Read the model definition and answer for the solid it produces. Units are mm, in the model's axes. A direction names the side the tool comes from. Coordinates: 2 decimals unless noted, no trailing zeros. Loops run counter-clockwise (first coordinate to the right, second up) from the corner with the lowest first, then second, coordinate; pieces in that order, holes last.
Q1. The mould has two halves that part along X. Classify faces 6 (the face through (-38.966, -1.985, -0.521)), 7 (the face through (9.028, 35.796, -19.907)), 8 (the face through (0, 36, -28)): pulls with the +X half, pulls with the -X half, needs draft (parallel to the pull), parting line crosses it, or undercut.
Q2. Section C-C (y = 30) is taken. Give the vertices of the cut face in (x, z), then the cut area to 3 significant figures.
Q3. Straight lines are drawn through the part: line 1 (X direction, y = -5.5, z = 0); line 2 (Y direction, x = 3, z = 23.5); line 3 (Z direction, x = 0, y = 7). For each, find the intervals that lie inside material, in ascending order.
Q4. Flat-ended cylindrical pins translate along their axes: P1, Ø4.5, axis at x = -35, z = 0, coming from the +Y side; P2, Ø6, axis at y = 15.5, z = 10, coming from the +X side (3 decimals); P3, Ø6, axis at x = 3, y = 13, coming from the -Z side; P4, Ø9, axis at x = -35, z = 0, coming from the -Y side. Find the tip coordinate at first contact, or state that the pin passes through.
Q5. Which of the six approach directions +Z, -Z, +X, -X, +Y, -Y give full straight-line access (tool end or side, diameter ignored) to faces 1 (the face through (-0.2, -5.563, -25.254)), 2 (the face through (-9.028, 35.796, 19.907)), 3 (the face through (-0.2, -5.563, 25.254)), 4 (the face through (-33, -4, -2)), 5 (the face through (-8.804, 39.715, -19.706))?
Q6. Section A-A (x = 0) is taken. Count the separate pieces of the cut face and the enclosed holes in it, then the cut area to 3 significant figures.
from build123d import *

# Parameters (mm, degrees)
SKETCH1_R                     = 6.25
SKETCH1_R_2                   = 20
SKETCH1_R_3                   = 15
SKETCH1_R_4                   = 1.55
BOSS_EXTRUDE1_DEPTH           = 10
SKETCH1_3_R                   = 20
SKETCH1_3_R_2                 = 15
BOSS_EXTRUDE2_DEPTH           = 40
BOSS_EXTRUDE3_START           = 40
SKETCH1_4_R                   = 1.55
BOSS_EXTRUDE3_DEPTH           = 7.5
CBORE_FOR_M4_SHCS1_AT_2_COUNT = 2
CBORE_FOR_M4_SHCS1_AT_2_PITCH = 70
FILLET1_R                     = 25
FILLET3_R                     = 4
FILLET2_R                     = 1


with BuildPart() as part:
    # Sketch1 → Boss-Extrude1 (new body)
    with BuildSketch(Plane(origin=(0, 0, 0), x_dir=(1, 0, 0), z_dir=(0, 1, 0))):
        with Locations((-35, 0)):
            Circle(SKETCH1_R)
        with BuildLine():
            Line((0, 30), (-38.386505715, 5.253006667))
            ThreePointArc((-38.386505715, 5.253006667), (-32.008609079, 5.487629758), (-28.75, 0))
            ThreePointArc((-28.75, 0), (-32.008609079, -5.487629758), (-38.386505715, -5.253006667))
            Line((-38.386505715, -5.253006667), (0, -30))
            Line((0, -30), (-14.90711985, -13.333333333))
            ThreePointArc((-14.90711985, -13.333333333), (-20, 0), (-14.90711985, 13.333333333))
            Line((-14.90711985, 13.333333333), (0, 30))
        make_face()
        Circle(SKETCH1_R_2)
        Circle(SKETCH1_R_3, mode=Mode.SUBTRACT)
        with BuildLine():
            Line((14.90711985, 13.333333333), (0, 30))
            Line((0, 30), (-14.90711985, 13.333333333))
            ThreePointArc((-14.90711985, 13.333333333), (0, 20), (14.90711985, 13.333333333))
        make_face()
        with Locations((0, 24.13)):
            Circle(SKETCH1_R_4, mode=Mode.SUBTRACT)
        with Locations((0, 24.13)):
            Circle(SKETCH1_R_4)
        with BuildLine():
            Line((38.386505715, 5.253006667), (0, 30))
            Line((0, 30), (14.90711985, 13.333333333))
            ThreePointArc((14.90711985, 13.333333333), (18.683447179, 7.136441795), (20, 0))
            ThreePointArc((20, 0), (18.683447179, -7.136441795), (14.90711985, -13.333333333))
            Line((14.90711985, -13.333333333), (0, -30))
            Line((0, -30), (38.386505715, -5.253006667))
            ThreePointArc((38.386505715, -5.253006667), (28.75, 0), (38.386505715, 5.253006667))
        make_face()
        with BuildLine():
            Line((-14.90711985, -13.333333333), (0, -30))
            Line((0, -30), (14.90711985, -13.333333333))
            ThreePointArc((14.90711985, -13.333333333), (0, -20), (-14.90711985, -13.333333333))
        make_face()
        with Locations((0, -24.13)):
            Circle(SKETCH1_R_4, mode=Mode.SUBTRACT)
        with Locations((0, -24.13)):
            Circle(SKETCH1_R_4)
        with Locations((35, 0)):
            Circle(SKETCH1_R)
    extrude(amount=-BOSS_EXTRUDE1_DEPTH)

    # Sketch1<3> → Boss-Extrude2 (add)
    with BuildSketch(Plane(origin=(0, 0, 0), x_dir=(1, 0, 0), z_dir=(0, 1, 0))):
        Circle(SKETCH1_3_R)
        Circle(SKETCH1_3_R_2, mode=Mode.SUBTRACT)
    extrude(amount=BOSS_EXTRUDE2_DEPTH)

    # Sketch1<4> → Boss-Extrude3 (add)
    with BuildSketch(Plane(origin=(0, 0, 0), x_dir=(1, 0, 0), z_dir=(0, 1, 0)).offset(BOSS_EXTRUDE3_START)):
        with BuildLine():
            Line((14.90711985, 13.333333333), (0, 30))
            Line((0, 30), (-14.90711985, 13.333333333))
            ThreePointArc((-14.90711985, 13.333333333), (0, 20), (14.90711985, 13.333333333))
        make_face()
        with Locations((0, 24.13)):
            Circle(SKETCH1_4_R, mode=Mode.SUBTRACT)
        with BuildLine():
            Line((-14.90711985, -13.333333333), (0, -30))
            Line((0, -30), (14.90711985, -13.333333333))
            ThreePointArc((14.90711985, -13.333333333), (0, -20), (-14.90711985, -13.333333333))
        make_face()
        with Locations((0, -24.13)):
            Circle(SKETCH1_4_R, mode=Mode.SUBTRACT)
    extrude(amount=-BOSS_EXTRUDE3_DEPTH)

    # Sketch3 → CBORE for M4 SHCS1 (revolve, cut)
    with BuildSketch(Plane(origin=(-35, 0, 0), x_dir=(0, 0, 1), z_dir=(1, 0, 0))):
        Polygon((0, 0), (0, 11.442065486), (2.4, 10), (2.4, 4), (4, 4), (4, 0.025), (4.025, 0), align=None)
    cbore_for_m4_shcs1 = revolve(axis=Axis((-35, 6.35, 0), (0, -1, 0)), mode=Mode.SUBTRACT)

    # CBORE for M4 SHCS1 at 2: CBORE for M4 SHCS1 ×2
    with Locations(*[(i * CBORE_FOR_M4_SHCS1_AT_2_PITCH, 0, 0) for i in range(1, CBORE_FOR_M4_SHCS1_AT_2_COUNT)]):
        add(cbore_for_m4_shcs1, mode=Mode.SUBTRACT)

    # Fillet1
    fillet1_edges = [part.edges().sort_by_distance(p)[0] for p in [
        (0, -5, -30),
        (0, -5, 30),
    ]]
    fillet(fillet1_edges, radius=FILLET1_R)

    # Fillet3
    fillet3_edges = [part.edges().sort_by_distance(p)[0] for p in [
        (0, 36.25, -30),
        (0, 36.25, 30),
    ]]
    fillet(fillet3_edges, radius=FILLET3_R)

    # Fillet2
    fillet2_edges = [part.edges().sort_by_distance(p)[0] for p in [
        (41.25, 0, 0),
        (-25.966264287, 0, 13.260081708),
        (-20, 0, 0),
        (-20, 40, 0),
        (-8.94427191, 40, -20),
        (8.94427191, 40, -20),
        (18.683447179, 40, 7.136441795),
        (8.94427191, 40, 20),
        (-8.94427191, 40, 20),
        (25.966264287, 0, -13.260081708),
        (25.966264287, 0, 13.260081708),
        (0, 0, 25.25513008),
        (0, 0, -25.25513008),
        (-41.25, 0, 0),
        (0, 40, 28),
        (0, 40, -28),
        (-25.966264287, 0, -13.260081708),
    ]]
    fillet(fillet2_edges, radius=FILLET2_R)


solid = part.part
Numbers:
1. face 6: undercut
1. face 7: pulls with the +X half
1. face 8: parting line crosses it
2. outline: circle Ø40 at (0, 0); hole circle Ø30 at (0, 0)
2. area: 550 mm2
3. line 1: x = -41.25 to -37.4, -32.6 to -15, 15 to 32.6, 37.4 to 41.25
3. line 2: y = -10 to 0, 32.5 to 40
3. line 3: z = -20 to -15, 15 to 20
4. P1: passes through
4. P2: stops at x = 18.735
4. P3: stops at z = -20
4. P4: stops at y = -10
5. face 1: -Z, -Y
5. face 2: +Z, -X, +Y
5. face 3: +Z, -Y
5. face 4: +Y
5. face 5: -Z, -X, +Y
6. separate pieces: 4
6. enclosed holes: 0
6. area: 678 mm2
